Here's how the part is built. I have some questions about the finished solid (model axes, mm). Face numbers are marked on the shaded views. Coordinates: 2 decimals unless noted, no trailing zeros. Write each loop counter-clockwise with the first axis right and the second up, starting at its lowest first coordinate (ties: lowest second). Pieces come first, ordered by that corner, then holes.
Item 1: I'm going to push flat-ended pins straight in: pin 1 Ø5 at (x, y) = (0.5, 22) entering from +Z; pin 2 Ø2 at (x, y) = (2.5, 5.5) entering from -Z. Where does each tip first touch, or does it pass through?
Item 2: If we section it at C-C (y = 18.5): Please give me the cut outline in (x, z), then the cut area to 3 significant figures.
Item 3: If I drill on line 1 (Z direction, x = -0.25, y = 25); line 2 (Y direction, x = 9.25, z = 1.45); line 3 (X direction, y = 43, z = 1.2), over which ranges is the centre line in solid material (lowest first)?
Item 4: We'd pull the mould along Z, two halves only. Please class the marked faces 1, 2, 3 and 4: +Z half, -Z half, draft (parallel to the pull), parting line (faces both ways), or undercut.
Item 5: If we section it at A-A (x = 18.5): Please give me the cut outline in (y, z), then the cut area to 3 significant figures.
Item 6: If we section it at B-B (z = -1.5): Please give me the cut outline in (x, y).
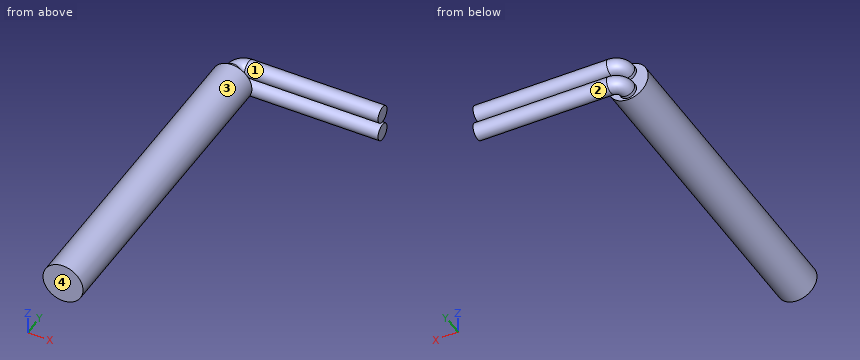
from build123d import *

# Parameters (mm, degrees)
SKETCH1_R           = 3
BOSS_EXTRUDE1_DEPTH = 47
SKETCH3_R           = 1.25


with BuildPart() as part:
    # Sketch1 → Boss-Extrude1 (new body)
    with BuildSketch(Plane(origin=(0, 0, 0), x_dir=(1, 0, 0), z_dir=(0, 1, 0))):
        with Locations(Location((0, 0, 0), (0, 0, 270))):
            Circle(SKETCH1_R)
    extrude(amount=BOSS_EXTRUDE1_DEPTH)

    # Sweep1: sweep along a path in Sketch2
    with BuildLine(Plane.XY.offset(1.5)) as sweep1_path:
        Line((0, 47), (0, 47.5))
        ThreePointArc((0, 47.5), (0.439339828, 48.560660172), (1.5, 49))
        Line((1.5, 49), (21.5, 49))
    # Sketch3 → Sweep1 (sweep)
    with BuildSketch(Plane(origin=(0, 47, 0), x_dir=(1, 0, 0), z_dir=(0, 1, 0))):
        with Locations((0, -1.5)):
            Circle(SKETCH3_R)
    sweep1 = sweep(path=sweep1_path.line)

    # Mirror1: Sweep1 across plane
    add(sweep1.mirror(Plane.XY))


solid = part.part
Answer list:
1. pin 1: stops at z = 3
1. pin 2: stops at z = -2.6
2. outline: circle Ø6 at (0, 0)
2. area: 28.3 mm2
3. line 1: z = -2.99 to 2.99
3. line 2: y = 47.75 to 50.25
3. line 3: x = -2.75 to 2.75
4. face 1: undercut
4. face 2: undercut
4. face 3: parting line
4. face 4: draft
5. outline: circle Ø2.5 at (49, -1.5); circle Ø2.5 at (49, 1.5)
5. area: 9.82 mm2
6. outline: (-2.6, 0) - (2.6, 0) - (2.6, 47) - (1.25, 47) - (1.25, 47.5) arc R0.25 cw to (1.5, 47.75) - (21.5, 47.75) - (21.5, 50.25) - (1.5, 50.25) arc R2.75 ccw to (-1.25, 47.5) - (-1.25, 47) - (-2.6, 47) - close
